The listing builds one solid part. Answer for the finished solid, in the listing's coordinates (mm). A direction names the side the tool comes from. Round coordinates to 2 decimals unless told otherwise and drop trailing zeros. Order: outer loops, then holes, each group sorted by start corner. A loop starts at its lowest first (then second) coordinate and runs counter-clockwise, first axis right, second up. Notation, with made-up numbers: (44, 41.5) - (65, 41.5) arc R28 ccw to (65, 60.5) - close; hole circle Ø1 at (11.25, 32). An arc over 180 degrees is marked (long way). Use CSV: the item, a comma, the result in double quotes. Start each with the question number.
Item 1: Straight lines are drawn through the part: line 1 along X through (y, z) = (-69, 36.5); line 2 along Y through (x, z) = (-9, 11); line 3 along Z through (x, y) = (15.5, -60). For each, find the intervals that lie inside material, in ascending order. Write a range as [from, to].
Item 2: Find section C-C, the plane y = -18. Give the vertices of the cut face in (x, z).
Item 3: Find section D-D, the plane z = 36.5. Give the vertices of the cut face in (x, y).
Item 4: Find section A-A, the plane z = 30.5. Give the vertices of the cut face in (x, y).
Item 5: Find section B-B, the plane x = -22.5. Give the vertices of the cut face in (y, z), plus the area to 3 significant figures.
Item 6: Determine the mould class of faces 4 (the flat face through (-30, -37, 2)), 5 (the flat face through (0, -70, 25)), 6 (the flat face through (-3, -75, 22)) for opening direction Y: +Y half, -Y half, draft (parallel to the pull), parting line (faces both ways), or undercut.
Item 7: For faces 1 (the flat face through (-29, -37, 4)), 2 (the cylindrical face through (-22.465, -48.056, 43.54)), 3 (the flat face through (0, -37, 5)), determine the directions among +Z, -Z, +X, -X, +Y, -Y from which every point of the face is accessible in a straight line to the end or side of a thin tool.
Item 8: Flat-ended cylindrical pins translate along their axes: P1, Ø10, axis at y = -41.5, z = 6.5, coming from the -X side; P2, Ø6, axis at y = -46.5, z = 31.5, coming from the -X side; P3, Ø1.8, axis at x = -26.5, y = -46.5, coming from the +Z side; P4, Ø0.5, axis at x = -29, y = -29.5, coming from the +Z side. Find the tip coordinate at first contact, or state that the pin passes through.
```python
from build123d import *

# Parameters (mm, degrees)
F1_DEPTH = 75
F2_R     = 0.5
F3_W     = 50
F3_H     = 40
F4_DEPTH = 75
F5_T     = -5
F6_R     = 10
F7_DEPTH = 50
F8_R     = 2


with BuildPart() as f1:
    # F0 (on Front) → F1 (new body)
    with BuildSketch(Plane.XZ):
        Polygon((25, 4), (-25, 4), (-25, 2.3), (-25, 0), (25, 0), align=None)
        Polygon((-25, 0), (-25, 2.3), (-28.2, 2.3), (-28.2, 4), (-30, 4), (-30, 0), align=None)
    extrude(amount=F1_DEPTH)

    # F2
    f2_edges = [f1.edges().sort_by_distance(p)[0] for p in [
        (-25, -37.5, 2.3),
        (-28.2, -37.5, 2.3),
    ]]
    fillet(f2_edges, radius=F2_R)

    # F3 (on Front) → F4 (join)
    with BuildSketch(Plane.XZ):
        with Locations((0, 24)):
            Rectangle(F3_W, F3_H)
    extrude(amount=F4_DEPTH)

    # F5
    f5_openings = [f1.faces().sort_by_distance(p)[0] for p in [
        (0, -37.5, 44),
    ]]
    offset(amount=F5_T, openings=f5_openings)

    # F6 (on face) → F7 (cut, through all)
    with BuildSketch(Plane(origin=(-25, 0, 0), x_dir=(0, -1, 0), z_dir=(-1, 0, 0))):
        with Locations((37.5, 44)):
            Circle(F6_R)
    extrude(amount=-F7_DEPTH, mode=Mode.SUBTRACT)

    # F8
    f8_edges = [f1.edges().sort_by_distance(p)[0] for p in [
        (22.5, -47.5, 44),
        (-22.5, -47.5, 44),
        (-22.5, -27.5, 44),
        (22.5, -27.5, 44),
    ]]
    fillet(f8_edges, radius=F8_R)


solid = f1.part
```
Worked out:
1,line 1,"x = [-25, -20], [20, 25]"
1,line 2,"y = [-75, -70], [-5, 0]"
1,line 3,"z = [0, 5]"
2,outline,"(-30, 0) - (25, 0) - (25, 44) - (20, 44) - (20, 5) - (-20, 5) - (-20, 44) - (-25, 44) - (-25, 2.8) arc R0.5 cw to (-25.5, 2.3) - (-27.7, 2.3) arc R0.5 cw to (-28.2, 2.8) - (-28.2, 4) - (-30, 4) - close"
3,outline,"(-25, -75) - (25, -75) - (25, -44.11) - (20, -44.11) - (20, -70) - (-20, -70) - (-20, -44.11) - (-25, -44.11) - close; (-25, -30.89) - (-20, -30.89) - (-20, -5) - (20, -5) - (20, -30.89) - (25, -30.89) - (25, 0) - (-25, 0) - close"
4,outline,"(-25, -75) - (25, -75) - (25, 0) - (-25, 0) - close; hole (-20, -70) - (20, -70) - (20, -5) - (-20, -5) - close"
5,outline,"(-75, 0) - (0, 0) - (0, 44) - (-25.67, 44) arc R2 ccw to (-27.64, 42.33) arc R10 cw to (-47.36, 42.33) arc R2 ccw to (-49.33, 44) - (-75, 44) - close"
5,area,"3,140 mm²"
6,face 4,"draft"
6,face 5,"undercut"
6,face 6,"-Y half"
7,face 1,"+Z, -X, +Y, -Y"
7,face 2,"+Z, +X, -X"
7,face 3,"+Z"
8,P1,"stops at x = -30"
8,P2,"stops at x = -25"
8,P3,"stops at z = 2.3"
8,P4,"stops at z = 4"
